Study the drawing (mm; zero at the part's minimum x, y, z) and answer. Round coordinates to 2 decimals unless told otherwise and drop trailing zeros. Loops run counter-clockwise (first coordinate to the right, second up) from the corner with the lowest first, then second, coordinate; pieces in that order, holes last. Notation, with made-up numbers: (84, 19.25) -> (139, 19.25) arc R27 cw to (139, 36.25) -> close; hole circle Ø4 at (15, 2.25). An arc over 180 degrees is marked (long way). Answer in a Markdown table with one row per item. Add a question column.
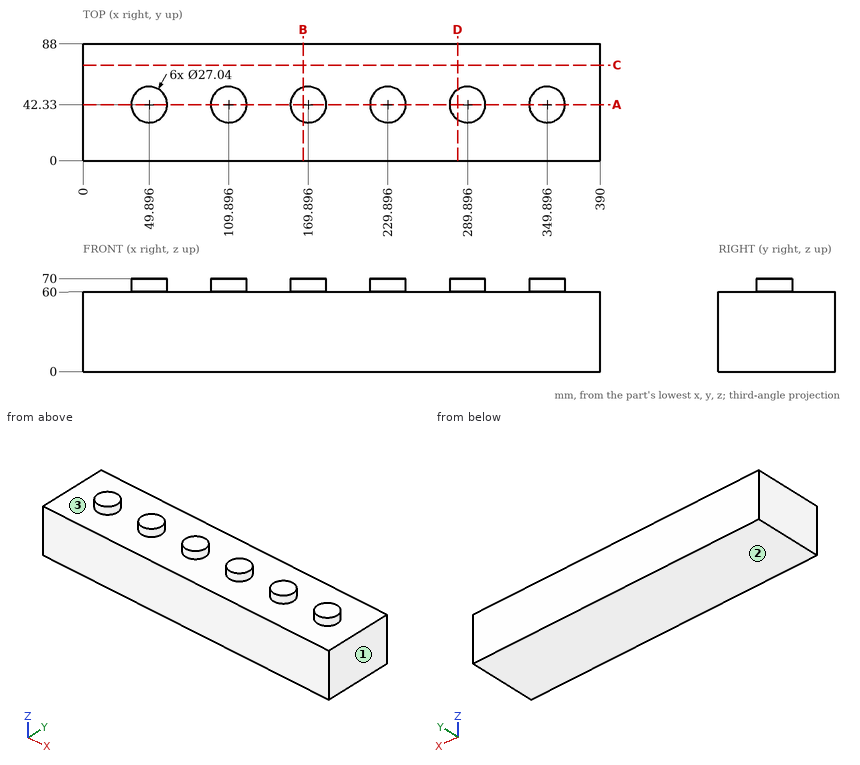
Item 1: A flat-ended cylindrical pin translates along its axis: P1, Ø5, axis at x = 174.5, y = 10.5, coming from the -Z side. Find the tip coordinate at first contact, or state that the pin passes through.
Item 2: Section C-C, the plane y = 72 is taken. Write down the section's boundary in (x, z).
Item 3: Consider L1, parallel to Z at x = 242, y = 21.5. Determine where the line is inside the solid, lowest interval first. Write a range as from..to.
Item 4: Section B-B, the plane x = 166 is taken. Write down the section's boundary in (y, z).
Item 5: Section A-A, the plane y = 42.33 is taken. Write down the section's boundary in (x, z) (1 decimal), and give its area (3 significant figures).
Item 6: Section D-D, the plane x = 282.5 is taken. Write down the section's boundary in (y, z).
Item 7: The mould has two halves that part along X. Classify the marked faces 1, 2 and 3: +X half, -X half, draft (parallel to the pull), parting line (faces both ways), or undercut.
Here are the results:
| question | item | result |
|---|---|---|
| 1 | P1 | stops at z = 0 |
| 2 | outline | (0, 0) -> (390, 0) -> (390, 60) -> (0, 60) -> close |
| 3 | L1 | z = 0..60 |
| 4 | outline | (0, 0) -> (88, 0) -> (88, 60) -> (55.28, 60) -> (55.28, 70) -> (29.38, 70) -> (29.38, 60) -> (0, 60) -> close |
| 5 | outline | (0, 0) -> (390, 0) -> (390, 60) -> (363.4, 60) -> (363.4, 70) -> (336.4, 70) -> (336.4, 60) -> (303.4, 60) -> (303.4, 70) -> (276.4, 70) -> (276.4, 60) -> (243.4, 60) -> (243.4, 70) -> (216.4, 70) -> (216.4, 60) -> (183.4, 60) -> (183.4, 70) -> (156.4, 70) -> (156.4, 60) -> (123.4, 60) -> (123.4, 70) -> (96.4, 70) -> (96.4, 60) -> (63.4, 60) -> (63.4, 70) -> (36.4, 70) -> (36.4, 60) -> (0, 60) -> close |
| 5 | area | 25,000 mm² |
| 6 | outline | (0, 0) -> (88, 0) -> (88, 60) -> (53.65, 60) -> (53.65, 70) -> (31.01, 70) -> (31.01, 60) -> (0, 60) -> close |
| 7 | face 1 | +X half |
| 7 | face 2 | draft |
| 7 | face 3 | undercut |
